from build123d import *

# Parameters (mm, degrees)
BASE_FLANGE1_DEPTH = 60
SKETCH6_R          = 5
SKETCH6_R_2        = 2.5
CUT_EXTRUDE1_DEPTH = 212.187120819
CUT_EXTRUDE2_DEPTH = 10
FILLET1_R          = 7


# Sheet-metal steps are written as plain solids
with BuildPart() as part:
    # Sketch1 → Base-Flange1 (new body)
    with BuildSketch(Plane(origin=(0, 0, 0), x_dir=(0, 0, -1), z_dir=(1, 0, 0))):
        with BuildLine():
            Line((-95, 70), (-95, 8))
            ThreePointArc((-95, 8), (-92.656854249, 2.343145751), (-87, 0))
            Line((-87, 0), (87, 0))
            ThreePointArc((87, 0), (92.656854249, 2.343145751), (95, 8))
            Line((95, 8), (95, 70))
            Line((95, 70), (92, 70))
            Line((92, 70), (92, 8))
            ThreePointArc((92, 8), (90.535533906, 4.464466094), (87, 3))
            Line((87, 3), (-87, 3))
            ThreePointArc((-87, 3), (-90.535533906, 4.464466094), (-92, 8))
            Line((-92, 8), (-92, 70))
            Line((-92, 70), (-95, 70))
        make_face()
    extrude(amount=BASE_FLANGE1_DEPTH)

    # Sketch6 → Cut-Extrude1 (cut, through all)
    with BuildSketch(Plane.XY.offset(95)):
        with Locations((30, 50)):
            Circle(SKETCH6_R)
        with Locations((11.75, 50)):
            Circle(SKETCH6_R_2)
        with Locations((48.25, 50)):
            Circle(SKETCH6_R_2)
    extrude(amount=-CUT_EXTRUDE1_DEPTH, mode=Mode.SUBTRACT)

    # Sketch7 → Cut-Extrude2 (cut)
    with BuildSketch(Plane(origin=(0, 0, 0), x_dir=(-1, 0, 0), z_dir=(0, -1, 0))):
        with BuildLine():
            Line((-6, 70), (-6, -70))
            ThreePointArc((-6, -70), (-7.5, -71.5), (-9, -70))
            Line((-9, -70), (-9, 70))
            ThreePointArc((-9, 70), (-7.5, 71.5), (-6, 70))
        make_face()
        with BuildLine():
            Line((-54, 70), (-54, -70))
            ThreePointArc((-54, -70), (-52.5, -71.5), (-51, -70))
            Line((-51, -70), (-51, 70))
            ThreePointArc((-51, 70), (-52.5, 71.5), (-54, 70))
        make_face()
    extrude(amount=-CUT_EXTRUDE2_DEPTH, mode=Mode.SUBTRACT)

    # Fillet1
    fillet1_edges = [part.edges().sort_by_distance(p)[0] for p in [
        (0, 70, -93.5),
        (0, 70, 93.5),
        (60, 70, -93.5),
        (60, 70, 93.5),
    ]]
    fillet(fillet1_edges, radius=FILLET1_R)


solid = part.part
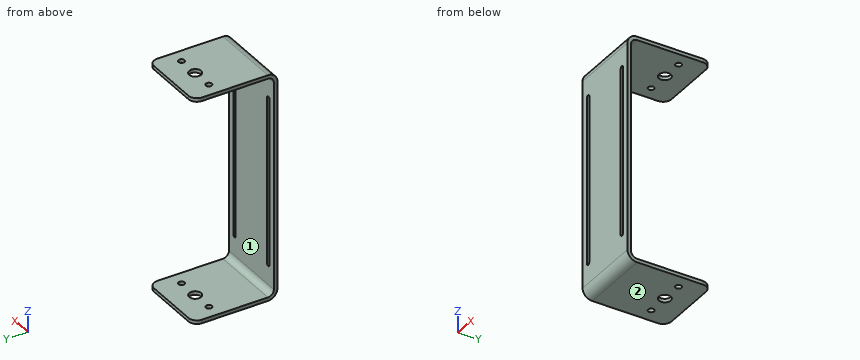
The listing builds one solid part. Answer for the finished solid, in the listing's coordinates (mm). Face numbers are marked on the shaded views. A direction names the side the tool comes from. Coordinates: 2 decimals unless noted, no trailing zeros. Loops run counter-clockwise (first coordinate to the right, second up) from the corner with the lowest first, then second, coordinate; pieces in that order, holes last. Notation, with made-up numbers: (84.25, 50.25) -> (129.25, 50.25) arc R28 cw to (129.25, 73.25) -> close; hole circle Ø3 at (-5.5, 27.5). An arc over 180 degrees is marked (long way). Answer in a Markdown table with one row per item. Add a question column.
1. The part is cut by section C-C, the plane y = 40. Write down the section's boundary in (x, z).
2. The part is cut by section D-D, the plane x = 39.5. Write down the section's boundary in (y, z).
3. For the marked faces 1 and 2, determine the directions among +Z, -Z, +X, -X, +Y, -Y from which every point of the face is accessible in a straight line to the end or side of a thin tool.
4. Consider line 1 (Z direction, x = 38, y = 62.5); line 2 (Y direction, x = 10.5, z = -44); line 3 (Y direction, x = 30, z = -94.15). Determine where each line is inside the solid, lowest interval first. Write a range as [from, to].
5. The part is cut by section A-A, the plane x = 48.25. Write down the section's boundary in (y, z).
6. The part is cut by section B-B, the plane z = -6. Write down the section's boundary in (x, y), then the cut area to 3 significant figures.
7. Flat-ended cylindrical pins translate along their axes: P1, Ø6, axis at x = 8, z = -51.5, coming from the +Y side; P2, Ø6.5, axis at x = 48.25, y = 50, coming from the +Z side; P3, Ø9, axis at x = 30, y = 50, coming from the -Z side. Find the tip coordinate at first contact, or state that the pin passes through.
Answer below:
| question | item | result |
|---|---|---|
| 1 | outline | (0, -95) -> (60, -95) -> (60, -92) -> (0, -92) -> close; (0, 92) -> (60, 92) -> (60, 95) -> (0, 95) -> close |
| 2 | outline | (0, -87) arc R8 ccw to (8, -95) -> (70, -95) -> (70, -92) -> (8, -92) arc R5 cw to (3, -87) -> (3, 87) arc R5 cw to (8, 92) -> (70, 92) -> (70, 95) -> (8, 95) arc R8 ccw to (0, 87) -> close |
| 3 | face 1 | +X, -X, +Y |
| 3 | face 2 | -Z, +X, -X, +Y, -Y |
| 4 | line 1 | [-95, -92], [92, 95] |
| 4 | line 2 | [0, 3] |
| 4 | line 3 | [4.41, 45], [55, 70] |
| 5 | outline | (0, -87) arc R8 ccw to (8, -95) -> (47.5, -95) -> (47.5, -92) -> (8, -92) arc R5 cw to (3, -87) -> (3, 87) arc R5 cw to (8, 92) -> (47.5, 92) -> (47.5, 95) -> (8, 95) arc R8 ccw to (0, 87) -> close; (52.5, -95) -> (70, -95) -> (70, -92) -> (52.5, -92) -> close; (52.5, 92) -> (70, 92) -> (70, 95) -> (52.5, 95) -> close |
| 6 | outline | (0, 0) -> (6, 0) -> (6, 3) -> (0, 3) -> close; (9, 0) -> (51, 0) -> (51, 3) -> (9, 3) -> close; (54, 0) -> (60, 0) -> (60, 3) -> (54, 3) -> close |
| 6 | area | 162 mm2 |
| 7 | P1 | y = 3 |
| 7 | P2 | z = 95 |
| 7 | P3 | through |
